Answer from the drawing. Dimensions are ordinates in mm from the lowest x, y and z of the part. A direction names the side the tool comes from. Round coordinates to 2 decimals unless told otherwise and drop trailing zeros. Write each loop counter-clockwise with the first axis right and the second up, starting at its lowest first coordinate (ties: lowest second). Pieces come first, ordered by that corner, then holes. Notation, with made-up numbers: M 74.25,87.25 L 105.25,87.25 A23 ccw 105.25,104.25 Z; hole C 41.25,42 d8. An arc over 180 degrees is marked long. Answer as CSV lines item,"result". Start each with the question number.
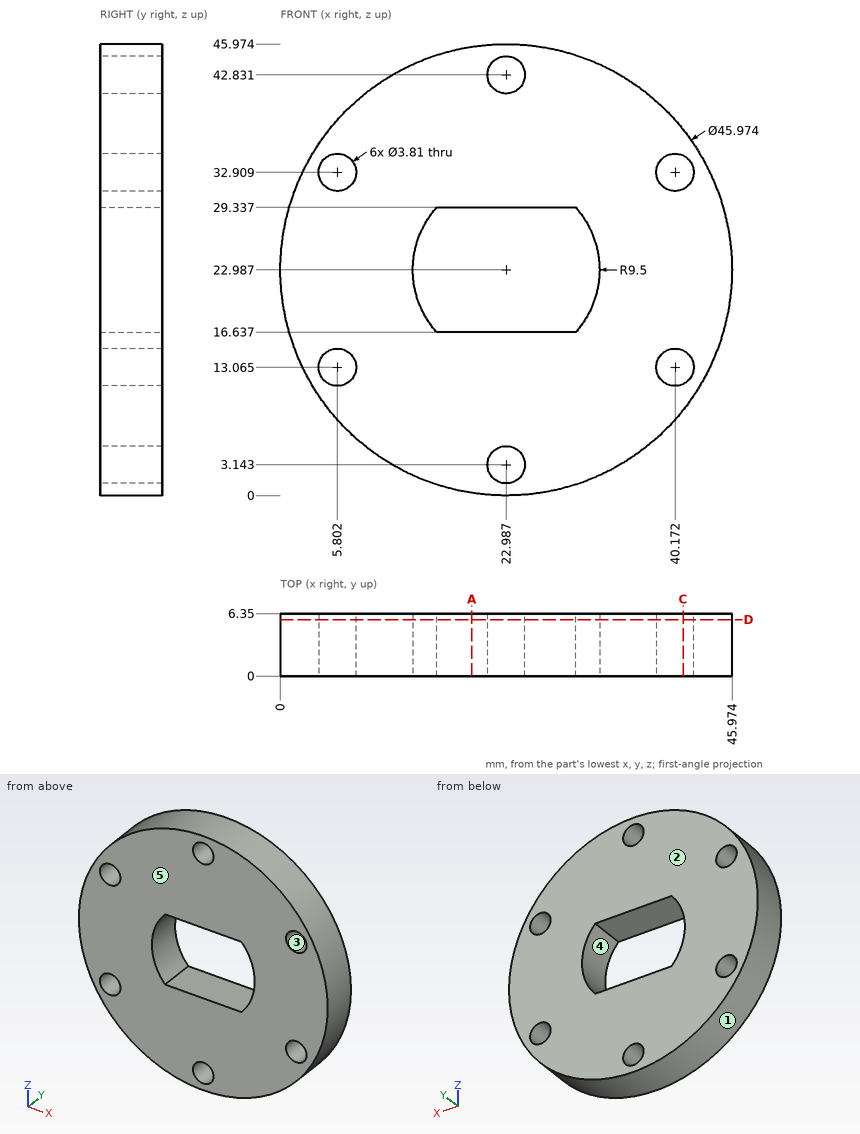
Q1. The mould has two halves that part along X. Classify the marked faces 1, 2 and 3: +X half, -X half, draft (parallel to the pull), parting line (faces both ways), or undercut.
Q2. Straight lines are drawn through the part: L1, parallel to Z at x = 7.5, y = 3.25 (1 decimal); L2, parallel to Z at x = 23.5, y = 3.5 (1 decimal); L3, parallel to X at y = 5.75, z = 32 (1 decimal). For each, find the intervals that lie inside material, in ascending order.
Q3. Find section A-A (x = 19.5). Determine the outline of the cut face in (y, z).
Q4. For the marked faces 4 and 5, determine the directions among +Z, -Z, +X, -X, +Y, -Y from which every point of the face is accessible in a straight line to the end or side of a thin tool.
Q5. Each of these flat-tipped pins is pushed along its axis until it touches: P1, Ø2, axis at y = 4, z = 35, coming from the -X side; P2, Ø1.9, axis at x = 22.5, y = 2, coming from the -Z side; P3, Ø3, axis at x = 8, y = 2.5, coming from the -Z side. Where does it stop, or does it pass through?
Q6. Find section C-C (x = 41). Count the separate pieces of the cut face and the enclosed holes in it, plus the area to 3 significant figures.
Q7. Find section D-D (y = 5.75). Determine the outline of the cut face in (x, z) (1 decimal).
Reported:
1,face 1,"parting line"
1,face 2,"draft"
1,face 3,"undercut"
2,L1,"z = 6 to 12.2, 13.9 to 32, 33.8 to 40"
2,L2,"z = 0 to 1.3, 5 to 16.6, 29.3 to 41, 44.7 to 46"
2,L3,"x = 1.8 to 4.1, 7.5 to 38.5, 41.8 to 44.1"
3,outline,"M 0,0.27 L 6.35,0.27 L 6.35,16.64 L 0,16.64 Z; M 0,29.34 L 6.35,29.34 L 6.35,45.71 L 0,45.71 Z"
4,face 4,"+Y, -Y"
4,face 5,"+Z, -Z, +X, -X, -Y"
5,P1,"stops at x = 2.81"
5,P2,"stops at z = 0"
5,P3,"stops at z = 4.37"
6,separate pieces,"3"
6,enclosed holes,"0"
6,area,"138 mm2"
7,outline,"C 23,23 d46; hole C 5.8,13.1 d3.8; hole C 5.8,32.9 d3.8; hole M 15.9,16.6 L 30.1,16.6 A9.5 ccw 30.1,29.3 L 15.9,29.3 A9.5 ccw Z; hole C 23,3.1 d3.8; hole C 23,42.8 d3.8; hole C 40.2,13.1 d3.8; hole C 40.2,32.9 d3.8"
